from build123d import *

# Parameters (mm, degrees)
SKETCH1_R                                       = 1.75
SKETCH1_R_2                                     = 6
BOSS_EXTRUDE1_DEPTH                             = 70
SKETCH2_W                                       = 36
SKETCH2_H                                       = 58
CUT_EXTRUDE1_DEPTH                              = 52
SKETCH3_W                                       = 60
SKETCH3_H                                       = 58
CUT_EXTRUDE2_DEPTH                              = 23
SKETCH4_R                                       = 21
CUT_EXTRUDE3_DEPTH                              = 2.5
FILLET2_R                                       = 5
FILLET3_R                                       = 3
SKETCH5_R                                       = 11.025
CUT_EXTRUDE4_DEPTH                              = 7
CBORE_FOR_M6_SOCKET_HEAD_CAP_SCREW1_D           = 7
CBORE_FOR_M6_SOCKET_HEAD_CAP_SCREW1_CBORE_D     = 11
CBORE_FOR_M6_SOCKET_HEAD_CAP_SCREW1_CBORE_DEPTH = 6
SKETCH8_W                                       = 59.674444403
SKETCH8_H                                       = 31.446844148
CUT_EXTRUDE5_DEPTH                              = 71.0000001
CUT_EXTRUDE6_DEPTH                              = 36
CUT_EXTRUDE6_DEPTH_BACK                         = 36
CHAMFER1_SIZE                                   = 1


with BuildPart() as part:
    # Sketch1 → Boss-Extrude1 (new body)
    with BuildSketch(Plane.XY):
        Polygon((-35, -74.75), (-35, 28.55), (35, 28.55), (35, -74.75), (23, -74.75), (23, -49.75), (-23, -49.75), (-23, -74.75), align=None)
        with Locations((-23.55, 23.55)):
            Circle(SKETCH1_R, mode=Mode.SUBTRACT)
        with Locations((23.55, -23.55)):
            Circle(SKETCH1_R, mode=Mode.SUBTRACT)
        with Locations((23.55, 23.55)):
            Circle(SKETCH1_R, mode=Mode.SUBTRACT)
        with Locations((-23.55, -23.55)):
            Circle(SKETCH1_R, mode=Mode.SUBTRACT)
        Circle(SKETCH1_R_2, mode=Mode.SUBTRACT)
    extrude(amount=BOSS_EXTRUDE1_DEPTH)

    # Sketch2 → Cut-Extrude1 (cut)
    with BuildSketch(Plane.XY.offset(70)):
        with Locations((0, -0.45)):
            Rectangle(SKETCH2_W, SKETCH2_H)
    extrude(amount=-CUT_EXTRUDE1_DEPTH, mode=Mode.SUBTRACT)

    # Sketch3 → Cut-Extrude2 (cut)
    with BuildSketch(Plane.XY.offset(70)):
        with Locations((0, -0.45)):
            Rectangle(SKETCH3_W, SKETCH3_H)
    extrude(amount=-CUT_EXTRUDE2_DEPTH, mode=Mode.SUBTRACT)

    # Sketch4 → Cut-Extrude3 (cut)
    with BuildSketch(Plane.XY.offset(47)):
        Circle(SKETCH4_R)
    extrude(amount=-CUT_EXTRUDE3_DEPTH, mode=Mode.SUBTRACT)

    # Fillet2
    fillet2_edges = [part.edges().sort_by_distance(p)[0] for p in [
        (35, -74.75, 35),
        (-35, -74.75, 35),
        (35, 28.55, 35),
        (-35, 28.55, 35),
        (18, -29.45, 32.5),
        (-18, -29.45, 32.5),
    ]]
    fillet(fillet2_edges, radius=FILLET2_R)

    # Fillet3
    fillet3_edges = [part.edges().sort_by_distance(p)[0] for p in [
        (23, -49.75, 35),
        (-23, -49.75, 35),
        (30, -29.45, 58.5),
        (-30, -29.45, 58.5),
    ]]
    fillet(fillet3_edges, radius=FILLET3_R)

    # Sketch5 → Cut-Extrude4 (cut)
    with BuildSketch(Plane.XY.offset(18)):
        Circle(SKETCH5_R)
    extrude(amount=-CUT_EXTRUDE4_DEPTH, mode=Mode.SUBTRACT)

    # CBORE for M6 Socket Head Cap Screw1 (through all)
    with Locations(Plane(origin=(0, -29.45, 0), x_dir=(1, 0, 0), z_dir=(0, 1, 0))):
        with Locations((0, -28.5), (-19.75, -58.5), (12, -58.5)):
            CounterBoreHole(CBORE_FOR_M6_SOCKET_HEAD_CAP_SCREW1_D / 2, CBORE_FOR_M6_SOCKET_HEAD_CAP_SCREW1_CBORE_D / 2, CBORE_FOR_M6_SOCKET_HEAD_CAP_SCREW1_CBORE_DEPTH)

    # Sketch8 → Cut-Extrude5 (cut, through all)
    with BuildSketch(Plane.XY.offset(70)):
        with Locations((-33.952701125, -65.473422074)):
            Rectangle(SKETCH8_W, SKETCH8_H)
    extrude(amount=-CUT_EXTRUDE5_DEPTH, mode=Mode.SUBTRACT)

    # Sketch9 → Cut-Extrude6 (cut, two sides)
    with BuildSketch(Plane(origin=(0, 0, 0), x_dir=(0, 0, -1), z_dir=(1, 0, 0))) as cut_extrude6_sk:
        Polygon((-47, 28.55), (-70, 28.55), (-70, -29.45), align=None)
    extrude(amount=CUT_EXTRUDE6_DEPTH, mode=Mode.SUBTRACT)
    extrude(cut_extrude6_sk.sketch, amount=-CUT_EXTRUDE6_DEPTH_BACK, mode=Mode.SUBTRACT)

    # Chamfer1
    chamfer1_edges = [part.edges().sort_by_distance(p)[0] for p in [
        (-6, 0, 11),
    ]]
    chamfer(chamfer1_edges, length=CHAMFER1_SIZE)


solid = part.part
The model under review builds one solid part; all positions refer to its coordinate system, in mm. A direction names the side the tool comes from. Round coordinates to 2 decimals unless told otherwise and drop trailing zeros. Loops run counter-clockwise (first coordinate to the right, second up) from the corner with the lowest first, then second, coordinate; pieces in that order, holes last. Notation, with made-up numbers: (-28, -9.75) -> (18, -9.75) arc R16 cw to (18, -4.75) -> close; hole circle Ø4 at (16.5, -20). An arc over 180 degrees is marked (long way). Write item = value, one per line. Start each with the question number.
Item 1: Take a section at C-C on z = 58.5. Count the separate pieces of the cut face and the enclosed holes in it, plus the area to 3 significant figures.
Item 2: Insertion check: pin 1 (2.5 mm diameter, centred on x = -20, y = -4, fed in from +Z); pin 2 (3 mm diameter, centred on x = -23.55, y = -23.55, fed in from -Z); pin 3 (17.5 mm diameter, centred on x = 12, z = 58.5, fed in from -Y); pin 4 (18.5 mm diameter, centred on x = -25.5, y = -7, fed in from +Z). Each pin has a flat end and moves straight along its axis. Give the tip position at first contact, or say it passes through.
Item 3: For faces 4 (the cylindrical face through (16.57, -27.95, 32.3)), 5 (the flat face through (-16, -35.45, 58)), 6 (the flat face through (-7, -49.75, 35)), 7 (the cylindrical face through (21, 0, 46)), list the 3-axis set-ups (+Z, -Z, +X, -X, +Y, -Y) from which the entire face can be reached by the end or side of a thin tool; tool diameter is ignored.
Item 4: Take a section at B-B on x = 0. Give the boundary of the cut face in (y, z) (3 decimals), plus the area to 3 significant figures.
Item 5: To check wall thickness, follow L1, parallel to X at y = 23.5, z = 7; L2, parallel to Y at x = -23.55, z = 32; L3, parallel to X at y = -23.55, z = 23. State the ranges of each line that lie inside material, in increasing order.
Item 6: Take a section at A-A on z = 8. Give the boundary of the cut face in (x, y).
Item 7: Mouldability with a two-part tool opening along Y and no side actions: class faces 1 (the flat face through (27, -74.75, 35)), 2 (the cylindrical face through (-6, 0, 5)), 3 (the cylindrical face through (11.284, -32.408, 53.047)) as released by +Y, released by -Y, zero draft, split by the parting line, or undercut.
Item 8: Take a section at D-D on x = -19.75. Give the boundary of the cut face in (y, z).
Result:
q1.separate_pieces = 3
q1.enclosed_holes = 0
q1.area = 1,680 mm²
q2.pin_1 = 47
q2.pin_2 = through
q2.pin_3 = -49.85
q2.pin_4 = 64.3
q3.face_4 = +Z, +Y
q3.face_5 = +Y
q3.face_6 = +Z, -Z, -X, -Y
q3.face_7 = +Z
q4.outline = (-49.75, 0) -> (-6, 0) -> (-6, 10) -> (-7, 11) -> (-11.025, 11) -> (-11.025, 18) -> (-29.45, 18) -> (-29.45, 23) -> (-35.45, 23) -> (-35.45, 25) -> (-49.75, 25) -> close; (-49.75, 32) -> (-35.45, 32) -> (-35.45, 34) -> (-29.45, 34) -> (-29.45, 70) -> (-49.75, 70) -> close; (6, 0) -> (28.55, 0) -> (28.55, 18) -> (11.025, 18) -> (11.025, 11) -> (7, 11) -> (6, 10) -> close
q4.area = 2,010 mm²
q5.L1 = -35 to -25.3, -21.8 to 21.8, 25.3 to 35
q5.L2 = -49.75 to -25.3, -21.8 to 21.8, 25.3 to 28.55
q5.L3 = -35 to -25.3, -21.8 to -18, 18 to 21.8, 25.3 to 35
q6.outline = (-35, -49.75) -> (20, -49.75) arc R3 cw to (23, -52.75) -> (23, -74.75) -> (30, -74.75) arc R5 ccw to (35, -69.75) -> (35, 23.55) arc R5 ccw to (30, 28.55) -> (-30, 28.55) arc R5 ccw to (-35, 23.55) -> close; hole circle Ø3.5 at (-23.55, -23.55); hole circle Ø3.5 at (-23.55, 23.55); hole circle Ø12 at (0, 0); hole circle Ø3.5 at (23.55, -23.55); hole circle Ø3.5 at (23.55, 23.55)
q7.face_1 = released by -Y
q7.face_2 = undercut
q7.face_3 = zero draft
q8.outline = (-49.75, 0) -> (28.55, 0) -> (28.55, 47) -> (7.14, 47) -> (7.14, 44.5) -> (-7.14, 44.5) -> (-7.14, 47) -> (-29.45, 47) -> (-29.45, 53) -> (-35.45, 53) -> (-35.45, 55) -> (-49.75, 55) -> close; (-49.75, 62) -> (-35.45, 62) -> (-35.45, 64) -> (-29.45, 64) -> (-29.45, 70) -> (-49.75, 70) -> close
